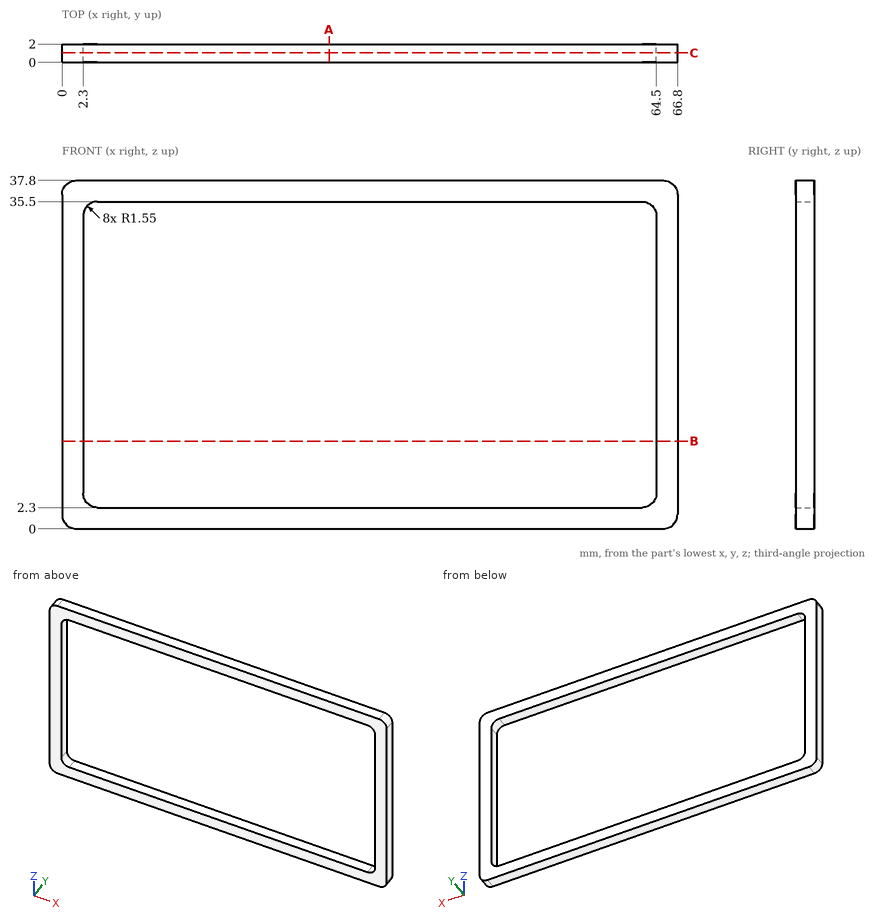
Source: three-view drawing plus pictorial views. Frame: mm from the lowest corner of the part. Round coordinates to 2 decimals unless told otherwise and drop trailing zeros. Loops run counter-clockwise (first coordinate to the right, second up) from the corner with the lowest first, then second, coordinate; pieces in that order, holes last. Notation, with made-up numbers: M 7.5,62.25 L 21.5,62.25 A23 cw 21.5,95.25 Z; hole C -35,-22 d10. An arc over 180 degrees is marked long. Put each result on its own line as item: value.
(1) Section C-C, the plane y = 1.05. Return loops of the section in (x, z), and give its area (3 significant figures).
Solutions:
outline: M 0,1.55 A1.55 ccw 1.55,0 L 65.25,0 A1.55 ccw 66.8,1.55 L 66.8,36.25 A1.55 ccw 65.25,37.8 L 1.55,37.8 A1.55 ccw 0,36.25 Z; hole M 2.3,3.85 A1.55 ccw 3.85,2.3 L 62.95,2.3 A1.55 ccw 64.5,3.85 L 64.5,33.95 A1.55 ccw 62.95,35.5 L 3.85,35.5 A1.55 ccw 2.3,33.95 Z
area: 460 mm²
(2) Ray query, line 1 (X direction, y = 0.6, z = 26); line 2 (Z direction, x = 48.5, y = 0.35); line 3 (Z direction, x = 3, y = 1.4). Return the intervals inside material, ascending. Write a range as [from, to].
Solutions:
line 1: [0, 2.3], [64.5, 66.8]
line 2: [0, 2.3], [35.5, 37.8]
line 3: [0, 2.55], [35.25, 37.8]
(3) Section A-A, the plane x = 29. Return loops of the section in (y, z).
Solutions:
outline: M 0,0 L 2,0 L 2,2.3 L 0,2.3 Z; M 0,35.5 L 2,35.5 L 2,37.8 L 0,37.8 Z
(4) Section B-B, the plane z = 9.5. Return loops of the section in (x, y), and give its area (3 significant figures).
Solutions:
outline: M 0,0 L 2.3,0 L 2.3,2 L 0,2 Z; M 64.5,0 L 66.8,0 L 66.8,2 L 64.5,2 Z
area: 9.20 mm²
